Answer from the drawing. Dimensions are ordinates in mm from the lowest x, y and z of the part. A direction names the side the tool comes from. Coordinates: 2 decimals unless noted, no trailing zeros. Loops run counter-clockwise (first coordinate to the right, second up) from the corner with the lowest first, then second, coordinate; pieces in that order, holes last. Notation, with made-up numbers: (86.5, 88) -> (106.5, 88) arc R12 cw to (106.5, 111) -> close; hole circle Ø7 at (36, 77.5). An arc over 180 degrees is marked (long way). Use a Markdown table: item, result.
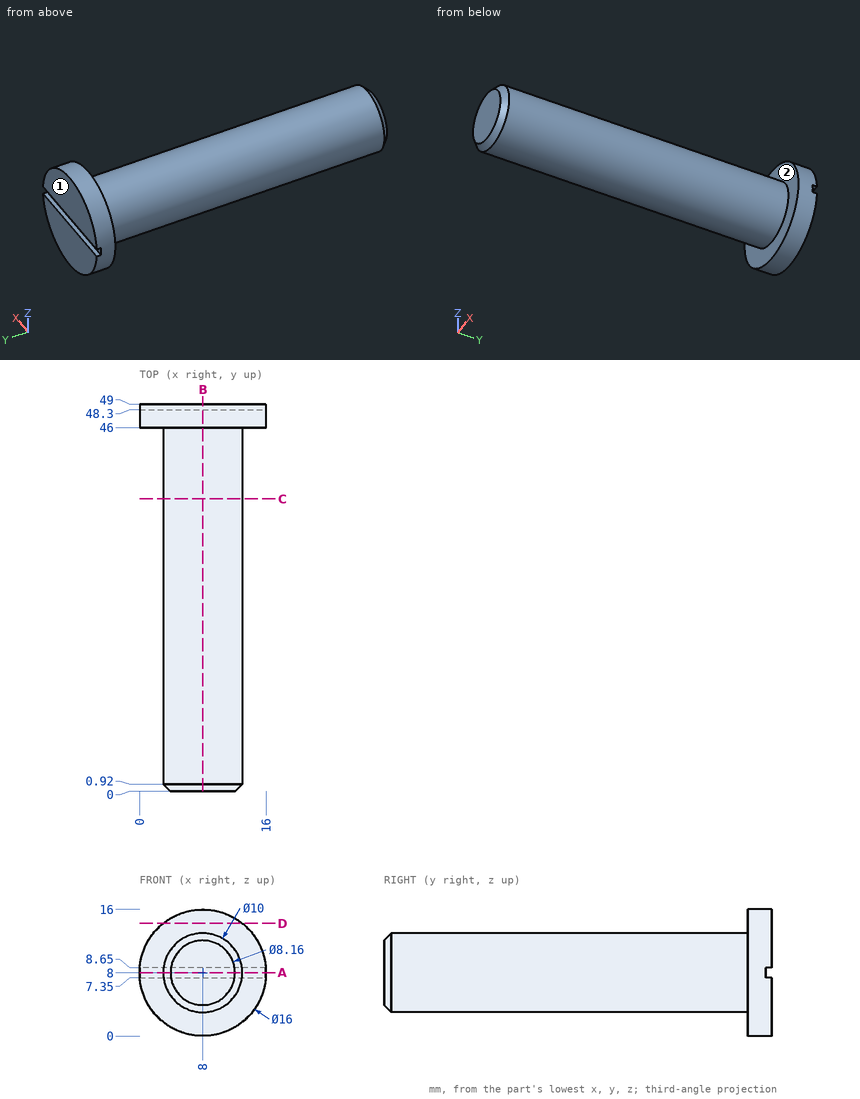
Q1. Section A-A on z = 8 is taken. Determine the outline of the cut face in (x, y), and give its area (3 significant figures).
Solved:
| item | result |
|---|---|
| outline | (0, 46) -> (3, 46) -> (3, 0.92) -> (3.92, 0) -> (12.08, 0) -> (13, 0.92) -> (13, 46) -> (16, 46) -> (16, 48.3) -> (0, 48.3) -> close |
| area | 496 mm² |
Q2. Section C-C on y = 37 is taken. Determine the outline of the cut face in (x, z), and give its area (3 significant figures).
Solved:
| item | result |
|---|---|
| outline | circle Ø10 at (8, 8) |
| area | 78.5 mm² |
Q3. Section D-D on z = 14.25 is taken. Determine the outline of the cut face in (x, y), and give its area (3 significant figures).
Solved:
| item | result |
|---|---|
| outline | (3.01, 46) -> (12.99, 46) -> (12.99, 49) -> (3.01, 49) -> close |
| area | 30.0 mm² |
Q4. Consider line 1 (Y direction, x = 8.25, z = 15.25); line 2 (Y direction, x = 11, z = 8.5); line 3 (X direction, y = 6, z = 10). Determine where each line is inside the solid, lowest interval first. Write a range as [from, to].
Solved:
| item | result |
|---|---|
| line 1 | [46, 49] |
| line 2 | [0, 48.3] |
| line 3 | [3.42, 12.58] |
Q5. Given pin 1 Ø1 at (x, z) = (11, 12.5) entering from -Y; pin 2 Ø4 at (y, z) = (19.5, 1.5) entering from +X; pin 3 Ø8 at (x, y) = (7.5, 32) entering from +Z, each flat-ended and moving along its own axis, determine where each tip first touches the part or whether it passes through.
Solved:
| item | result |
|---|---|
| pin 1 | y = 0.83 |
| pin 2 | x = 10.18 |
| pin 3 | z = 13 |
Q6. Section B-B on x = 8 is taken. Determine the outline of the cut face in (y, z).
Solved:
| item | result |
|---|---|
| outline | (0, 3.92) -> (0.92, 3) -> (46, 3) -> (46, 0) -> (49, 0) -> (49, 7.35) -> (48.3, 7.35) -> (48.3, 8.65) -> (49, 8.65) -> (49, 16) -> (46, 16) -> (46, 13) -> (0.92, 13) -> (0, 12.08) -> close |
Q7. For the marked faces 1 and 2, determine the directions among +Z, -Z, +X, -X, +Y, -Y from which every point of the face is accessible in a straight line to the end or side of a thin tool.
Solved:
| item | result |
|---|---|
| face 1 | +Z, -Z, +X, -X, +Y |
| face 2 | -Y |
